Check sheet for the modelled part. Datum: model origin and axes. Units: mm. Face numbers are marked on the shaded views. A direction names the side the tool comes from. Round coordinates to 2 decimals unless told otherwise and drop trailing zeros. Write each loop counter-clockwise with the first axis right and the second up, starting at its lowest first coordinate (ties: lowest second). Pieces come first, ordered by that corner, then holes. Notation, with made-up numbers: (-37, -16) -> (-4, -16) arc R15 cw to (-4, 5) -> close; hole circle Ø9 at (19.25, -11.5). An arc over 180 degrees is marked (long way). Write item = value, one per line.
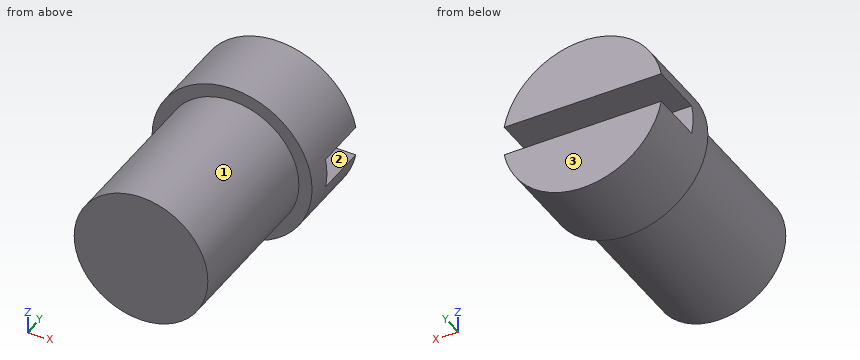
from build123d import *

# Parameters (mm, degrees)
SKETCH1_R           = 2.3749
BOSS_EXTRUDE1_DEPTH = 2.3622
SKETCH2_R           = 1.984375
BOSS_EXTRUDE2_DEPTH = 4.7625
SKETCH3_W           = 4.7498
SKETCH3_H           = 0.889
CUT_EXTRUDE1_DEPTH  = 1.5875


with BuildPart() as part:
    # Sketch1 → Boss-Extrude1 (new body)
    with BuildSketch(Plane(origin=(0, 0, 0), x_dir=(1, 0, 0), z_dir=(0, 1, 0))):
        Circle(SKETCH1_R)
    extrude(amount=BOSS_EXTRUDE1_DEPTH)

    # Sketch2 → Boss-Extrude2 (add)
    with BuildSketch(Plane(origin=(0, 0, 0), x_dir=(-1, 0, 0), z_dir=(0, -1, 0))):
        Circle(SKETCH2_R)
    extrude(amount=BOSS_EXTRUDE2_DEPTH)

    # Sketch3 → Cut-Extrude1 (cut)
    with BuildSketch(Plane(origin=(0, 2.3622, 0), x_dir=(1, 0, 0), z_dir=(0, 1, 0))):
        Rectangle(SKETCH3_W, SKETCH3_H)
    extrude(amount=-CUT_EXTRUDE1_DEPTH, mode=Mode.SUBTRACT)


solid = part.part
(1) Sectioned sample at B-B on x = 0. Enter the section's corners in (y, z).
Worked answers:
outline = (-4.76, -1.98) -> (0, -1.98) -> (0, -2.37) -> (2.36, -2.37) -> (2.36, -0.44) -> (0.77, -0.44) -> (0.77, 0.44) -> (2.36, 0.44) -> (2.36, 2.37) -> (0, 2.37) -> (0, 1.98) -> (-4.76, 1.98) -> close
(2) Sectioned sample at A-A on z = 0. Enter the section's corners in (x, y).
Worked answers:
outline = (-2.37, 0) -> (-1.98, 0) -> (-1.98, -4.76) -> (1.98, -4.76) -> (1.98, 0) -> (2.37, 0) -> (2.37, 0.77) -> (-2.37, 0.77) -> close
(3) Sectioned sample at C-C on y = -2.5. Enter the section's corners in (x, z), then the cut area to 3 significant figures.
Worked answers:
outline = circle Ø3.97 at (0, 0)
area = 12.4 mm²
(4) Access from +Z, -Z, +X, -X, +Y, -Y to the whole of each face (thin tool, end or side, straight path). Record for the marked faces 1, 2 and 3.
Worked answers:
face_1 = -Y
face_2 = +X, -X, +Y
face_3 = +Z, -Z, +X, -X, +Y
(5) Material ranges on L1, parallel to Y at x = -1.4, z = 1.8; L2, parallel to Z at x = 1, y = 1.5; L3, parallel to Y at x = 1.75, z = 0.25, recorded low to high. Write a range as [from, to].
Worked answers:
L1 = [0, 2.36]
L2 = [-2.15, -0.44], [0.44, 2.15]
L3 = [-4.76, 0.77]
(6) Go/stop test with flat-tipped pins: P1, Ø1.7, axis at x = 1, y = 1.5, coming from the -Z side; P2, Ø2, axis at x = 1, y = -4, coming from the -Z side; P3, Ø0.7, axis at x = 0, z = 0, coming from the +Y side. Record where each tip stops, or that it passes through.
Worked answers:
P1 = -2.37
P2 = -1.98
P3 = 0.77
(7) Sectioned sample at D-D on x = -1.3. Enter the section's corners in (y, z), then the cut area to 3 significant figures.
Worked answers:
outline = (-4.76, -1.5) -> (0, -1.5) -> (0, -1.99) -> (2.36, -1.99) -> (2.36, -0.44) -> (0.77, -0.44) -> (0.77, 0.44) -> (2.36, 0.44) -> (2.36, 1.99) -> (0, 1.99) -> (0, 1.5) -> (-4.76, 1.5) -> close
area = 22.3 mm²
